from build123d import *

# Parameters (mm, degrees)
BOSS_EXTRUDE2_DEPTH = 53.34
SKETCH4_R           = 1.7
CUT_EXTRUDE1_DEPTH  = 92.181462139
SKETCH5_R           = 1.65
CUT_EXTRUDE2_DEPTH  = 219.815917306
CUT_EXTRUDE3_REACH  = 101.921
SKETCH6_R           = 1.65548177
SKETCH6_R_2         = 1.651


with BuildPart() as part:
    # Sketch3 → Boss-Extrude2 (new body)
    with BuildSketch(Plane(origin=(0.39856693, 1.174139675, 38.425283804), x_dir=(0.9999462474151822, -0.00015834992252811985, -0.010367121374682776), z_dir=(0.010367121374682774, 0.030540538135663202, 0.999479763839562))):
        Polygon((35.811663947, 184.686461522), (70.101663947, 184.686461522), (70.101663947, 191.325794663), (50.92397302, 191.325794663), (40.119315635, 214.372267387), (-57.15, 214.372267387), (-57.15, 194.173966846), (-78.183444815, 173.140522031), (-72.925707516, 167.882784732), (-55.896794471, 184.911697776), (-45.736794471, 184.911697776), (-45.736794471, 210.086461522), (35.811663947, 210.086461522), align=None)
    extrude(amount=-BOSS_EXTRUDE2_DEPTH)

    # Sketch4 → Cut-Extrude1 (cut, through all)
    with BuildSketch(Plane(origin=(-0.030296425, 191.236544322, -5.843192728), x_dir=(0.999999987462651, 0.00015827605687458352, -4.836091908386067e-06), z_dir=(-0.0001583499225282815, 0.99953351642438, -0.030540538135663205))):
        with Locations(Location((55.718705533, -23.165573574, 0), (0, 0, 270))):
            Circle(SKETCH4_R)
        with Locations(Location((55.470585341, 0.766513873, 0), (0, 0, 270))):
            Circle(SKETCH4_R)
    extrude(amount=-CUT_EXTRUDE1_DEPTH, mode=Mode.SUBTRACT)

    # Sketch5 → Cut-Extrude2 (cut, through all)
    with BuildSketch(Plane(origin=(-125.675127332, 125.623262737, -2.535031563), x_dir=(-0.010088789926051056, 0.010084626405281995, 0.9998982531378351), z_dir=(-0.7071807426733389, 0.7068888977909322, -0.014264759791391517))):
        with Locations(Location((27.353288467, 72.760478035, 0), (0, 0, 270))):
            Circle(SKETCH5_R)
        with Locations(Location((17.431171, 84.018164474, 0), (0, 0, 90))):
            Circle(SKETCH5_R)
        with Locations(Location((2.224674143, 84.018164474, 0), (0, 0, 270))):
            Circle(SKETCH5_R)
        with Locations(Location((-7.697443324, 72.760478035, 0), (0, 0, 90))):
            Circle(SKETCH5_R)
    extrude(amount=-CUT_EXTRUDE2_DEPTH, mode=Mode.SUBTRACT)

    # Sketch6 → Cut-Extrude3 (cut, up to next)
    with BuildSketch(Plane(origin=(-0.033945832, 214.272266245, -6.547044407), x_dir=(0.999999987462651, 0.00015827605687420668, -4.836091908374553e-06), z_dir=(-0.00015834992252790448, 0.99953351642438, -0.030540538135663216)), mode=Mode.PRIVATE) as cut_extrude3_sk1:
        with Locations(Location((-43.266263609, 8.096604069, 0), (0, 0, 270))):
            Circle(SKETCH6_R)
    cut_extrude3_tool1 = extrude(cut_extrude3_sk1.sketch, amount=-CUT_EXTRUDE3_REACH, mode=Mode.PRIVATE) & part.part
    # Sketch6 → Cut-Extrude3 (cut, up to next)
    with BuildSketch(Plane(origin=(-0.033945832, 214.272266245, -6.547044407), x_dir=(0.999999987462651, 0.00015827605687420668, -4.836091908374553e-06), z_dir=(-0.00015834992252790448, 0.99953351642438, -0.030540538135663216)), mode=Mode.PRIVATE) as cut_extrude3_sk2:
        with Locations(Location((26.072009948, 8.815481008, 0), (0, 0, 270))):
            Circle(SKETCH6_R_2)
    cut_extrude3_tool2 = extrude(cut_extrude3_sk2.sketch, amount=-CUT_EXTRUDE3_REACH, mode=Mode.PRIVATE) & part.part
    # Sketch6 → Cut-Extrude3 (cut, up to next)
    with BuildSketch(Plane(origin=(-0.033945832, 214.272266245, -6.547044407), x_dir=(0.999999987462651, 0.00015827605687420668, -4.836091908374553e-06), z_dir=(-0.00015834992252790448, 0.99953351642438, -0.030540538135663216)), mode=Mode.PRIVATE) as cut_extrude3_sk3:
        with Locations(Location((26.493329766, -31.822334996, 0), (0, 0, 270))):
            Circle(SKETCH6_R_2)
    cut_extrude3_tool3 = extrude(cut_extrude3_sk3.sketch, amount=-CUT_EXTRUDE3_REACH, mode=Mode.PRIVATE) & part.part
    # Sketch6 → Cut-Extrude3 (cut, up to next)
    with BuildSketch(Plane(origin=(-0.033945832, 214.272266245, -6.547044407), x_dir=(0.999999987462651, 0.00015827605687420668, -4.836091908374553e-06), z_dir=(-0.00015834992252790448, 0.99953351642438, -0.030540538135663216)), mode=Mode.PRIVATE) as cut_extrude3_sk4:
        with Locations(Location((-42.844943791, -32.541211936, 0), (0, 0, 270))):
            Circle(SKETCH6_R_2)
    cut_extrude3_tool4 = extrude(cut_extrude3_sk4.sketch, amount=-CUT_EXTRUDE3_REACH, mode=Mode.PRIVATE) & part.part
    add(cut_extrude3_tool1.solids().sort_by_distance((-43.300209, 214.018144, -14.639662))[0], mode=Mode.SUBTRACT)
    add(cut_extrude3_tool2.solids().sort_by_distance((26.038064, 214.007163, -15.358539))[0], mode=Mode.SUBTRACT)
    add(cut_extrude3_tool3.solids().sort_by_distance((26.459384, 215.248331, 25.260318))[0], mode=Mode.SUBTRACT)
    add(cut_extrude3_tool4.solids().sort_by_distance((-42.878889, 215.259311, 25.979195))[0], mode=Mode.SUBTRACT)


solid = part.part
Geometry: final body of the model. Coordinates: model frame, mm. Round coordinates to 2 decimals unless told otherwise and drop trailing zeros. Order: outer loops, then holes, each group sorted by start corner. A loop starts at its lowest first (then second) coordinate and runs counter-clockwise, first axis right, second up. Notation, with made-up numbers: (28.25, 70) -> (80.25, 70) arc R23 ccw to (80.25, 95) -> close; hole circle Ø6 at (-8, 86.25). An arc over 180 degrees is marked (long way). Put each result on its own line as item: value. Start each with the question number.
Q1. Section D-D on x = 42.5. Return the cut outline in (y, z), and give its area (3 significant figures).
Q2. Line query: probe 1 along X at (y, z) = (186.5, 19); probe 2 along Y at (x, z) = (-41, 31); probe 3 along X at (y, z) = (211.5, 25.5). Output: solid intervals per line, ascending.
Q3. Section C-C on y = 189. Give the number of separate pieces and of enclosed holes in the cut face, and give its area (3 significant figures).
Q4. Pull-direction query (Z, two-part tool) for faces 1 (the cylindrical face through (-62.743, 183.738, 14.451)), 2 (the cylindrical face through (-62.5, 183.6, -0.2)); classes: +Z half, -Z half, draft (parallel to the pull), parting line (faces both ways), or undercut.
Q5. First-contact query: pin 1 (12 mm diameter, centred on x = 51.5, y = 177.5, fed in from -Z); pin 2 (6 mm diameter, centred on x = 22, z = 24.5, fed in from +Y); pin 3 (4 mm diameter, centred on y = 181, z = 2.5, fed in from -X); pin 4 (1.5 mm diameter, centred on y = 179.5, z = 13.5, fed in from +X). Flat tips, straight axial feed; report the tip coordinate or a pass-through.
Q6. Section B-B on z = 5. Return the cut outline in (x, y).
Q7. Section A-A on y = 200.5. Return the cut outline in (x, z), and give its area (3 significant figures).
Ans:
1. outline: (184.14, -20.97) -> (208.33, -21.71) -> (211.14, 31.57) -> (185.77, 32.35) -> close
1. area: 1,320 mm2
2. probe 1: x = -65.26 to -45.51, 36.04 to 54.93, 56.45 to 70.33
2. probe 2: y = 211.13 to 215.41
2. probe 3: x = -56.86 to -44.42, -41.34 to 24.81, 28.11 to 42.18
3. separate pieces: 2
3. enclosed holes: 2
3. area: 2,710 mm2
4. face 1: undercut
4. face 2: undercut
5. pin 1: passes through
5. pin 2: stops at y = 215.32
5. pin 3: stops at x = -72.42
5. pin 4: stops at x = -60.88
6. outline: (-78.11, 173.36) -> (-72.85, 168.1) -> (-55.82, 185.14) -> (-45.66, 185.14) -> (-45.65, 210.33) -> (35.9, 210.34) -> (35.89, 184.93) -> (70.19, 184.94) -> (70.19, 191.58) -> (51.01, 191.58) -> (40.21, 214.63) -> (-57.07, 214.62) -> (-57.07, 194.41) -> close
7. outline: (-57.33, -20.43) -> (-45.92, -20.55) -> (-45.37, 32.81) -> (-56.78, 32.93) -> close; (35.62, -21.4) -> (46.17, -21.51) -> (47.49, 31.85) -> (36.18, 31.96) -> close
7. area: 1,190 mm2
